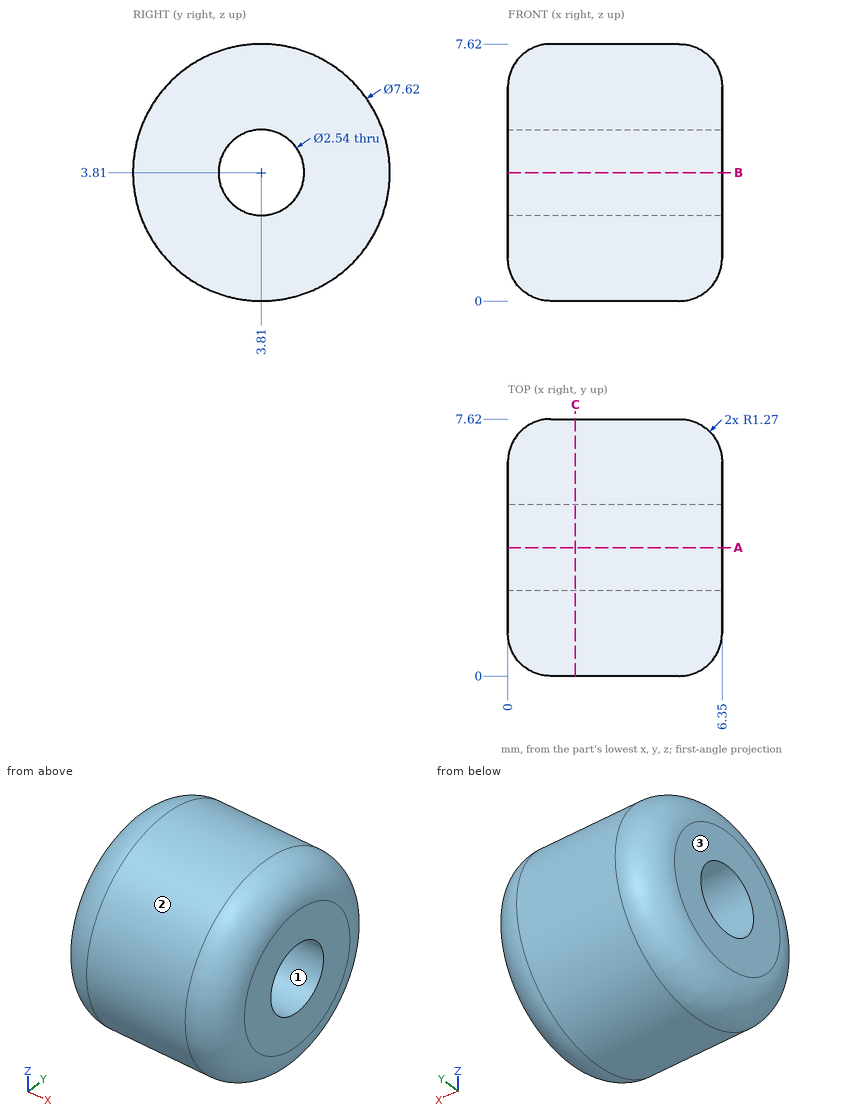
Input: dimensioned drawing with shaded views. Units: mm. Origin: part minimum x, y, z. Coordinates: 2 decimals unless noted, no trailing zeros. Order: outer loops, then holes, each group sorted by start corner. A loop starts at its lowest first (then second) coordinate and runs counter-clockwise, first axis right, second up.
(1) Section query C-C (x = 2). Return the cut outline in (y, z), plus the area to 3 significant figures.
(2) Material intervals for probe 1 along Z at (x, y) = (3.5, 3.81); probe 2 along Y at (x, z) = (3.75, 3); probe 3 along Y at (x, z) = (1, 3.25), sorted ascending.
(3) Section query A-A (y = 3.81). Return the cut outline in (x, z).
(4) First-contact query: pin 1 (1.5 mm diameter, centred on x = 1, y = 4.5, fed in from +Z). Flat tip, straight axial feed; report the tip coordinate or a pass-through.
(5) Draft query along Y for the marked faces 1, 2 and 3. Return one class per face: pulls with the +Y half, pulls with the -Y half, needs draft (parallel to the pull), parting line crosses it, or undercut.
Solution:
1. outline: circle Ø7.62 at (3.81, 3.81); hole circle Ø2.54 at (3.81, 3.81)
1. area: 40.5 mm2
2. probe 1: z = 0 to 2.54, 5.08 to 7.62
2. probe 2: y = 0.09 to 2.83, 4.79 to 7.53
2. probe 3: y = 0.07 to 2.67, 4.95 to 7.55
3. outline: (0, 1.27) arc R1.27 ccw to (1.27, 0) - (5.08, 0) arc R1.27 ccw to (6.35, 1.27) - (6.35, 2.54) - (0, 2.54) - close; (0, 5.08) - (6.35, 5.08) - (6.35, 6.35) arc R1.27 ccw to (5.08, 7.62) - (1.27, 7.62) arc R1.27 ccw to (0, 6.35) - close
4. pin 1: stops at z = 7.62
5. face 1: undercut
5. face 2: parting line crosses it
5. face 3: needs draft
